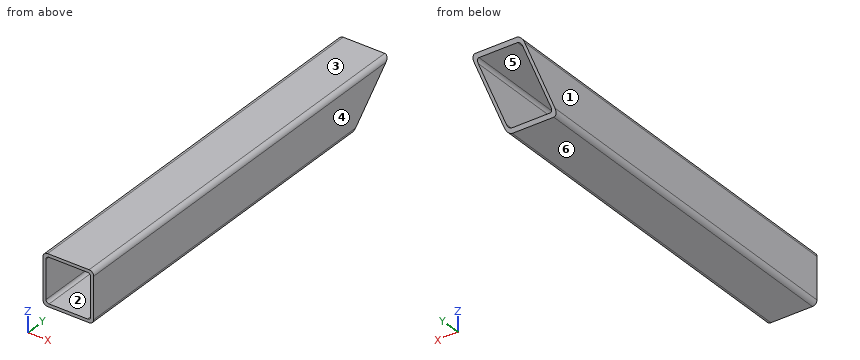
```python
from build123d import *

# Parameters (mm, degrees)
F1_DEPTH = 400
F3_DEPTH = 50.001


# Not quite as in the source:
# - a feature names something its author has since deleted; it is built from what else it names


with BuildPart() as f1:
    # F0 (on Front) → F1 (new body)
    with BuildSketch(Plane.XZ):
        with BuildLine():
            Line((45.5, 0), (4.5, 0))
            ThreePointArc((4.5, 0), (1.3180194847, -1.3180194847), (0, -4.5))
            Line((0, -4.5), (0, -45.5))
            ThreePointArc((0, -45.5), (1.3180194847, -48.6819805153), (4.5, -50))
            Line((4.5, -50), (45.5, -50))
            ThreePointArc((45.5, -50), (48.6819805153, -48.6819805153), (50, -45.5))
            Line((50, -45.5), (50, -4.5))
            ThreePointArc((50, -4.5), (48.6819805153, -1.3180194847), (45.5, 0))
        make_face()
        with BuildLine():
            ThreePointArc((3, -6), (3.8786796564, -3.8786796564), (6, -3))
            Line((6, -3), (44, -3))
            ThreePointArc((44, -3), (46.1213203436, -3.8786796564), (47, -6))
            Line((47, -6), (47, -44))
            ThreePointArc((47, -44), (46.1213203436, -46.1213203436), (44, -47))
            Line((44, -47), (6, -47))
            ThreePointArc((6, -47), (3.8786796564, -46.1213203436), (3, -44))
            Line((3, -44), (3, -6))
        make_face(mode=Mode.SUBTRACT)
    extrude(amount=F1_DEPTH)

    # F2 (on Right) → F3 (cut, through all)
    with BuildSketch(Plane.YZ):
        Polygon((29.2893218813, 0), (0, 0), (-45.5, -45.5), (-70.7106781187, -70.7106781187), (29.2893218813, -70.7106781187), align=None)
    extrude(amount=F3_DEPTH, mode=Mode.SUBTRACT)


solid = f1.part
```
Work out the finished part from the listing and answer in its coordinate system (mm). Face numbers are marked on the shaded views. A direction names the side the tool comes from. Round coordinates to 2 decimals unless told otherwise and drop trailing zeros. Write each loop counter-clockwise with the first axis right and the second up, starting at its lowest first coordinate (ties: lowest second). Pieces come first, ordered by that corner, then holes.
1) A cutting plane is placed at C-C on y = -86. Determine the outline of the cut face in (x, z).
2) Determine the mould class of the marked faces 3, 4, 5 and 6 for opening direction Z: pulls with the +Z half, pulls with the -Z half, needs draft (parallel to the pull), parting line crosses it, or undercut.
3) A cutting plane is placed at A-A on z = -16.5. Determine the outline of the cut face in (x, y).
4) Consider probe 1 along Z at (x, y) = (10, -108); probe 2 along X at (y, z) = (-62, -40.5); probe 3 along X at (y, z) = (-359.5, -45). Determine where each line is inside the solid, lowest interval first.
5) Which of the six approach directions +Z, -Z, +X, -X, +Y, -Y give full straight-line access (tool end or side, diameter ignored) to the marked faces 1 and 2?
6) A cutting plane is placed at B-B on x = 16.5. Determine the outline of the cut face in (y, z).
Entries:
1. outline: (0, -45.5) arc R4.5 ccw to (4.5, -50) - (45.5, -50) arc R4.5 ccw to (50, -45.5) - (50, -4.5) arc R4.5 ccw to (45.5, 0) - (4.5, 0) arc R4.5 ccw to (0, -4.5) - close; hole (3, -44) arc R3 ccw to (6, -47) - (44, -47) arc R3 ccw to (47, -44) - (47, -6) arc R3 ccw to (44, -3) - (6, -3) arc R3 ccw to (3, -6) - close
2. face 3: pulls with the +Z half
2. face 4: needs draft
2. face 5: undercut
2. face 6: pulls with the -Z half
3. outline: (0, -400) - (3, -400) - (3, -16.5) - (0, -16.5) - close; (47, -400) - (50, -400) - (50, -16.5) - (47, -16.5) - close
4. probe 1: z = -50 to -47, -3 to 0
4. probe 2: x = 0 to 3, 47 to 50
4. probe 3: x = 0 to 3.17, 46.83 to 50
5. face 1: +Z, -Z, -X, +Y, -Y
5. face 2: +Y, -Y
6. outline: (-400, -50) - (-50, -50) - (-47, -47) - (-400, -47) - close; (-400, -3) - (-3, -3) - (0, 0) - (-400, 0) - close
